```python
from build123d import *

# Parameters (mm, degrees)
F0_R     = 15.875
F0_R_2   = 9.525
F1_DEPTH = 25.4
F4_DEPTH = 50.8
F5_DEPTH = 25.4


with BuildPart() as f1:
    # F0 (on Front) → F1 (new body)
    with BuildSketch(Plane.XZ):
        Circle(F0_R)
        Circle(F0_R_2, mode=Mode.SUBTRACT)
    extrude(amount=F1_DEPTH)

    # F2 (on Right) → F3 (revolve)
    with BuildSketch(Plane.YZ):
        Polygon((-25.4, 27.556808), (-25.4, 15.875), (-12.7, 15.875), (-12.7, 42.56691), (-19.509828, 42.56691), (-20.829493, 42.56691), (-25.4, 37.756736), (-25.4, 33.107586), align=None)
        Polygon((-12.7, 42.56691), (-12.7, 15.875), (0, 15.875), (0, 27.556808), (0, 33.107586), (0, 37.756736), (-1.200963, 48.91691), (-4.570507, 42.56691), (-5.890172, 42.56691), align=None)
        Polygon((0, 33.107586), (0, 27.556808), (5.08, 33.107586), align=None)
        Polygon((0, 33.107586), (5.08, 33.107586), (0, 37.756736), align=None)
        Polygon((-30.48, 33.107586), (-25.4, 27.556808), (-25.4, 33.107586), align=None)
        Polygon((-30.48, 33.107586), (-25.4, 33.107586), (-25.4, 37.756736), align=None)
        Polygon((-24.199037, 48.91691), (-25.4, 37.756736), (-20.829493, 42.56691), align=None)
        Polygon((-20.829493, 42.56691), (-19.509828, 42.56691), (-19.509828, 55.26691), align=None)
        Polygon((-19.509828, 42.56691), (-12.7, 42.56691), (-12.7, 68.114896), align=None)
        Polygon((-12.7, 68.114896), (-12.7, 42.56691), (-5.890172, 42.56691), align=None)
        Polygon((-5.890172, 55.26691), (-5.890172, 42.56691), (-4.570507, 42.56691), align=None)
    revolve(axis=Axis((0, 0, 0), (0, 1, 0)))

    # F0 (on Front) → F4 (join)
    with BuildSketch(Plane.XZ):
        Circle(F0_R)
        Circle(F0_R_2, mode=Mode.SUBTRACT)
    extrude(amount=F4_DEPTH)

    # F0 (on Front) → F5 (join)
    with BuildSketch(Plane.XZ):
        Circle(F0_R)
        Circle(F0_R_2, mode=Mode.SUBTRACT)
    extrude(amount=-F5_DEPTH)


solid = f1.part
```
Geometry: final body of the model. Coordinates: model frame, mm. A direction names the side the tool comes from. Round coordinates to 2 decimals unless told otherwise and drop trailing zeros. Order: outer loops, then holes, each group sorted by start corner. A loop starts at its lowest first (then second) coordinate and runs counter-clockwise, first axis right, second up. Notation, with made-up numbers: M -1.5,28.5 L 48.5,28.5 A35 ccw 48.5,66.5 Z; hole C 38,-30 d10. An arc over 180 degrees is marked long. Use one line per item in the form item = value. Start each with the question number.
Q1. Mould query, pull axis X, two halves, no side actions, for faces 1 (the face through (7, 25.4, -7)), 2 (the face through (8.358, -25.647, 26.541)), 3 (the face through (-32.541, -30.233, -7.226)). Classes: +X half, -X half, draft (parallel to the pull), parting line (faces both ways), or undercut.
Q2. Access query for faces 4 (the face through (-41.94, -21.04, -9.31)), 5 (the face through (-12, 0, -12)), 6 (the face through (12, -25.4, -12)), 7 (the face through (7, -50.8, -7)). Directions: +Z, -Z, +X, -X, +Y, -Y. A direction counts if a zero-diameter tool reaches every point of the face in a straight line with its end or side. Return the directions, or none.
Q3. Pin query (flat end, axial travel): pin 1 Ø1.5 at (x, z) = (-53, 1) entering from +Y; pin 2 Ø11.5 at (x, z) = (0, 0) entering from +Y; pin 3 Ø8 at (x, z) = (-46, -1.5) entering from -Y. Return the tip coordinate at first contact, or that it passes through.
Q4. Cut plane D-D (y = -17.5). Return loops of the section in (x, z) (3 decimals), and give its area (3 significant figures).
Q5. Cut plane A-A (y = -46). Return loops of the section in (x, z) (3 decimals).
Q6. Cut plane B-B (x = -46). Count the separate pieces of the cut face and the enclosed holes in it, and give its area (3 significant figures).
Q7. Material intervals for line 1 (Z direction, x = 0, y = 9.75) (3 decimals); line 2 (Y direction, x = 41, z = 19); line 3 (Y direction, x = 45, z = -1.5), sorted ascending. Write a range as [from, to].
Geometry results:
q1.face_1 = draft
q1.face_2 = undercut
q1.face_3 = parting line
q2.face_4 = none
q2.face_5 = +Y
q2.face_6 = -Y
q2.face_7 = +Z, -Z, +X, -X, -Y
q3.pin_1 = -5.58
q3.pin_2 = through
q3.pin_3 = -24.94
q4.outline = C 0,0 d100.214; hole C 0,0 d19.05
q4.area = 7,600 mm^2
q5.outline = C 0,0 d31.75; hole C 0,0 d19.05
q6.separate_pieces = 5
q6.enclosed_holes = 0
q6.area = 917 mm^2
q7.line_1 = [-15.875, -9.525], [9.525, 15.875]
q7.line_2 = [-24.6, -22.22], [-20.56, -19.51], [-18.81, -6.59], [-5.89, -4.84], [-3.18, -0.8]
q7.line_3 = [-24.62, -22.13], [-20.57, -19.51], [-18.85, -6.55], [-5.89, -4.83], [-3.27, -0.78]
